from build123d import *

# Parameters (mm, degrees)
SKETCH3_W               = 25.4
SKETCH3_H               = 3.175
CUT_EXTRUDE1_DEPTH      = 13.7
CUT_EXTRUDE1_DEPTH_BACK = 13.7


with BuildPart() as part:
    # Sketch2 → Revolve1 (revolve)
    with BuildSketch(Plane(origin=(0, 0, 0), x_dir=(1, 0, 0), z_dir=(0, 1, 0))):
        Polygon((6.35, 7.9375), (6.35, 12.7), (445.226359817, 12.7), (445.226359817, 9.525), (521.426359817, 9.525), (521.426359817, 0), (0, 0), (0, 7.9375), align=None)
    revolve(axis=Axis((0, 0, 0), (1, 0, 0)))

    # Sketch3 → Cut-Extrude1 (cut, two sides)
    with BuildSketch(Plane(origin=(0, 0, 0), x_dir=(1, 0, 0), z_dir=(0, 1, 0))) as cut_extrude1_sk:
        with Locations((209.006359817, 11.1125)):
            Rectangle(SKETCH3_W, SKETCH3_H)
    extrude(amount=CUT_EXTRUDE1_DEPTH, mode=Mode.SUBTRACT)
    extrude(cut_extrude1_sk.sketch, amount=-CUT_EXTRUDE1_DEPTH_BACK, mode=Mode.SUBTRACT)


solid = part.part
Source: CAD feature listing. Evaluate the final solid. Frame: model axes, mm. A direction names the side the tool comes from. Round coordinates to 2 decimals unless told otherwise and drop trailing zeros. Loops run counter-clockwise (first coordinate to the right, second up) from the corner with the lowest first, then second, coordinate; pieces in that order, holes last. Notation, with made-up numbers: M -36.75,-34.75 L -31.75,-34.75 A8 cw -31.75,-19.75 Z; hole C 66.5,-5.75 d5. An arc over 180 degrees is marked long. Return JSON: item names as keys, results as strings. Group by question number.
1. Mould query, pull axis X, two halves, no side actions, for faces 1 (the face through (228.86, -12.4, 2.75)), 2 (the face through (0, 0, 0)), 3 (the face through (209, 0, -9.525)). Classes: released by +X, released by -X, zero draft, split by the parting line, or undercut.
2. Pin query (flat end, axial travel): pin 1 (6 mm diameter, centred on x = 81.5, y = 7.5, fed in from +Z); pin 2 (12.5 mm diameter, centred on y = 3.5, z = -0.5, fed in from -X); pin 3 (3 mm diameter, centred on x = 127.5, y = -3.5, fed in from +Z); pin 4 (5 mm diameter, centred on x = 137, y = -3, fed in from +Z). Return the tip coordinate at first contact, or that it passes through.
3. Section query C-C on x = 214. Output: boundary loops of the cut face in (y, z) (3 decimals).
4. Material intervals for line 1 along X through (y, z) = (1.75, -11); line 2 along X through (y, z) = (-9.25, 7); line 3 along Y through (x, z) = (361, 1.5), sorted ascending. Write a range as from..to.
5. Reachability of faces 4 (the face through (483.86, -5.796, 7.559)), 5 (the face through (521.426, 0, 0)), 6 (the face through (3.22, -7.75, 1.72)) from +Z, -Z, +X, -X, +Y, -Y: full face, straight path, thin tool, end or side. Return the list, or none.
6. Section query D-D on x = 59. Output: boundary loops of the cut face in (y, z), and give its area (3 significant figures).
Checks:
{
 "1": {"face 1": "zero draft", "face 2": "released by -X", "face 3": "undercut"},
 "2": {"pin 1": "stops at z = 11.88", "pin 2": "stops at x = 0", "pin 3": "stops at z = 12.54", "pin 4": "stops at z = 12.69"},
 "3": {"outline": "M -8.4,-9.525 L 8.4,-9.525 A12.7 ccw long Z"},
 "4": {"line 1": "x = 6.35..196.31, 221.71..445.23", "line 2": "x = 6.35..445.23", "line 3": "y = -12.61..12.61"},
 "5": {"face 4": "+X", "face 5": "+Z, -Z, +X, +Y, -Y", "face 6": "-X"},
 "6": {"outline": "C 0,0 d25.4", "area": "507 mm²"}
}
